Part model, mm, in its own coordinate system. A direction names the side the tool comes from. Give positions to 0.01 mm unless a question says otherwise; leave off trailing zeros. Loops run counter-clockwise (first coordinate to the right, second up) from the corner with the lowest first, then second, coordinate; pieces in that order, holes last. Notation, with made-up numbers: M 50.5,-30.5 L 79.5,-30.5 A17 ccw 79.5,-23.5 Z; hole C 23,-1 d10. An arc over 180 degrees is marked long. Answer in a Markdown table with one row per item.
from build123d import *

# Parameters (mm, degrees)
SKETCH1_R           = 30
SKETCH1_R_2         = 27
BOSS_EXTRUDE1_DEPTH = 160
SCALE1_SCALE        = 0.703703704
SKETCH3_R           = 25
BOSS_EXTRUDE4_DEPTH = 8


with BuildPart() as part:
    # Sketch1 → Boss-Extrude1 (new body)
    with BuildSketch(Plane.XY):
        Circle(SKETCH1_R)
        Circle(SKETCH1_R_2, mode=Mode.SUBTRACT)
    extrude(amount=BOSS_EXTRUDE1_DEPTH)


with BuildPart() as part_1:
    # Scale1: scaled about (0, 0, 0)
    add(part.part.scale(SCALE1_SCALE))

    # Sketch3 → Boss-Extrude4 (add)
    with BuildSketch(Plane.XY.offset(112.592592607)):
        Circle(SKETCH3_R)
    extrude(amount=BOSS_EXTRUDE4_DEPTH)


solid = part_1.part
(1) Which spindle directions (+Z, -Z, +X, -X, +Y, -Y) get a long thin tool onto all of the face, cutting with end or side? Do faces 1 (the face through (0, 0, 120.593)), 2 (the face through (-17, -13, 112.593)). Say none if no direction does.
Recorded:
| item | result |
|---|---|
| face 1 | +Z, +X, -X, +Y, -Y |
| face 2 | -Z |
(2) Saw through at A-A (x = 0). Write the cut outline in (y, z).
Recorded:
| item | result |
|---|---|
| outline | M -25,112.59 L -21.11,112.59 L -21.11,0 L -19,0 L -19,112.59 L 19,112.59 L 19,0 L 21.11,0 L 21.11,112.59 L 25,112.59 L 25,120.59 L -25,120.59 Z |
(3) Pull direction X, two halves, no side cores. Call faces 3 (the face through (23.846, 7.509, 116.537)), 4 (the face through (-19, 3, 0)), 5 (the face through (0, 0, 112.593)), 6 (the face through (-18.98, 0.84, 55.51)): +X half, -X half, draft (parallel to the pull), parting line (faces both ways), or undercut.
Recorded:
| item | result |
|---|---|
| face 3 | parting line |
| face 4 | draft |
| face 5 | undercut |
| face 6 | undercut |
(4) Saw through at B-B (z = 20.5). Write the cut outline in (x, y), plus the area to 3 significant figures.
Recorded:
| item | result |
|---|---|
| outline | C 0,0 d42.22; hole C 0,0 d38 |
| area | 266 mm^2 |
(5) Drill centre lines: line 1 along Y through (x, z) = (0, 30); line 2 along Z through (x, y) = (23, -7); line 3 along X through (y, z) = (13, 55). Where is each one in solid material? Low to high.
Recorded:
| item | result |
|---|---|
| line 1 | y = -21.11 to -19, 19 to 21.11 |
| line 2 | z = 112.59 to 120.59 |
| line 3 | x = -16.63 to -13.86, 13.86 to 16.63 |
(6) Pin check, flat tips, straight feed: pin 1 Ø5 at (x, z) = (-14, 32) entering from +Y; pin 2 Ø3 at (y, z) = (12, 13) entering from -X; pin 3 Ø1 at (y, z) = (-19, 85.5) entering from -X. Stop position of each tip, or through.
Recorded:
| item | result |
|---|---|
| pin 1 | stops at y = 17.7 |
| pin 2 | stops at x = -18.31 |
| pin 3 | stops at x = -10.17 |
